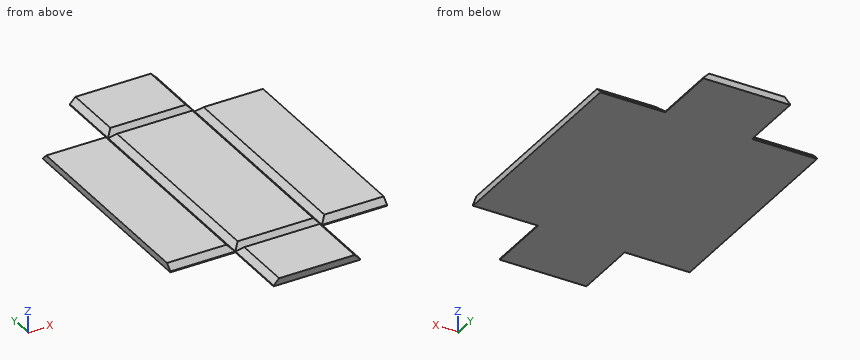
from build123d import *

# Parameters (mm, degrees)
SKETCH_W        = 20
SKETCH_H        = 50
SKETCH_W_2      = 15
SKETCH_H_2      = 15
PAD_DEPTH       = 1.5
POCKET_DEPTH    = 80.001
POCKET001_DEPTH = 50.001


with BuildPart() as part:
    # Sketch → Pad (new body)
    with BuildSketch(Plane.XY):
        Rectangle(SKETCH_W, SKETCH_H)
        with Locations((17.5, 0)):
            Rectangle(SKETCH_W_2, SKETCH_H)
        with Locations((-17.5, 0)):
            Rectangle(SKETCH_W_2, SKETCH_H)
        with Locations((0, 32.5)):
            Rectangle(SKETCH_W, SKETCH_H_2)
        with Locations((0, -32.5)):
            Rectangle(SKETCH_W, SKETCH_H_2)
    extrude(amount=PAD_DEPTH)

    # Sketch001 (on Face6 of Pad) → Pocket (cut, through all)
    with BuildSketch(Plane.XZ.offset(40)):
        Polygon((10, 0.2), (11.3, 1.5), (8.7, 1.5), align=None)
        Polygon((-11.3, 1.5), (-10, 0.2), (-8.7, 1.5), align=None)
    extrude(amount=-POCKET_DEPTH, mode=Mode.SUBTRACT)

    # Sketch002 (on Face10 of Pocket) → Pocket001 (cut, through all)
    with BuildSketch(Plane.YZ.offset(25)):
        Polygon((-25, 0.2), (-23.7, 1.5), (-26.3, 1.5), align=None)
        Polygon((25, 0.2), (26.3, 1.5), (23.7, 1.5), align=None)
    extrude(amount=-POCKET001_DEPTH, mode=Mode.SUBTRACT)


solid = part.part
For this review, take the finished solid that the model builds, in its own axes (mm). Give positions to 0.01 mm unless a question says otherwise; leave off trailing zeros. Loops run counter-clockwise (first coordinate to the right, second up) from the corner with the lowest first, then second, coordinate; pieces in that order, holes last.
Item 1: For line 1 along X through (y, z) = (12.5, 0.5); line 2 along Y through (x, z) = (-6, 0.6); line 3 along Y through (x, z) = (-7.5, 0.75), list the stretches that pass through material, from the lowest coordinate up.
Item 2: Take a section at D-D, the plane x = 13.5. State the section outline as (y, z) points, and give its area (3 significant figures).
Item 3: Take a section at A-A, the plane z = 0.45. State the section outline as (x, y) points, and give its area (3 significant figures).
Item 4: Take a section at B-B, the plane y = -10. State the section outline as (x, z) points, and give its area (3 significant figures).
Item 5: Take a section at C-C, the plane x = -0.5. State the section outline as (y, z) points, and give its area (3 significant figures).
Calculated:
1. line 1: x = -25 to -10.3, -9.7 to 9.7, 10.3 to 25
1. line 2: y = -40 to -25.4, -24.6 to 24.6, 25.4 to 40
1. line 3: y = -40 to -25.55, -24.45 to 24.45, 25.55 to 40
2. outline: (-25, 0) - (25, 0) - (25, 0.2) - (23.7, 1.5) - (-23.7, 1.5) - (-25, 0.2) - close
2. area: 73.3 mm2
3. outline: (-25, -24.75) - (-10.25, -24.75) - (-10.25, 24.75) - (-25, 24.75) - close; (-9.75, -40) - (9.75, -40) - (9.75, -25.25) - (-9.75, -25.25) - close; (-9.75, -24.75) - (9.75, -24.75) - (9.75, 24.75) - (-9.75, 24.75) - close; (-9.75, 25.25) - (9.75, 25.25) - (9.75, 40) - (-9.75, 40) - close; (10.25, -24.75) - (25, -24.75) - (25, 24.75) - (10.25, 24.75) - close
3. area: 3,000 mm2
4. outline: (-25, 0) - (25, 0) - (25, 1.5) - (11.3, 1.5) - (10, 0.2) - (8.7, 1.5) - (-8.7, 1.5) - (-10, 0.2) - (-11.3, 1.5) - (-25, 1.5) - close
4. area: 71.6 mm2
5. outline: (-40, 0) - (40, 0) - (40, 1.5) - (26.3, 1.5) - (25, 0.2) - (23.7, 1.5) - (-23.7, 1.5) - (-25, 0.2) - (-26.3, 1.5) - (-40, 1.5) - close
5. area: 117 mm2
